Read the model definition and answer for the solid it produces. Units are mm, in the model's axes. Coordinates: 2 decimals unless noted, no trailing zeros. Write each loop counter-clockwise with the first axis right and the second up, starting at its lowest first coordinate (ties: lowest second). Pieces come first, ordered by that corner, then holes.
1) The part is cut by section B-B (x = 0.55). Determine the outline of the cut face in (y, z), then the cut area to 3 significant figures.
2) Each of these flat-tipped pins is pushed along its axis until it touches: pin 1 Ø6.5 at (y, z) = (-17, -13) entering from +X; pin 2 Ø2.5 at (y, z) = (-8, -10) entering from -X. Where does it stop, or does it pass through?
3) Find the intervals of material crossed by line 1 (Y direction, x = 0.6, z = -13); line 2 (Y direction, x = 0.2, z = 10); line 3 (Z direction, x = 0.2, y = -5), in increasing order.
4) The part is cut by section A-A (y = -17). Determine the outline of the cut face in (x, z).
from build123d import *

# Parameters (mm, degrees)
SKETCH1_W                = 36
SKETCH1_H                = 120
BOSS_EXTRUDE1_DEPTH      = 1
F_4_0_4_DIAMETER_HOLE2_D = 4
F_4_0_4_DIAMETER_HOLE3_D = 4
BOSS_EXTRUDE2_DEPTH      = 1
FILLET1_R                = 4


with BuildPart() as part:
    # Sketch1 → Boss-Extrude1 (new body)
    with BuildSketch(Plane(origin=(0, 0, 0), x_dir=(0, 0, -1), z_dir=(1, 0, 0))):
        with Locations((0, -60)):
            Rectangle(SKETCH1_W, SKETCH1_H)
    extrude(amount=BOSS_EXTRUDE1_DEPTH)

    # Ø4.0 (4) Diameter Hole2 (through all)
    with Locations(Plane.ZY):
        with Locations((-10, -8), (10, -8)):
            Hole(F_4_0_4_DIAMETER_HOLE2_D / 2)

    # Ø4.0 (4) Diameter Hole3 (through all)
    with Locations(Plane.ZY):
        with Locations((-13, -17), (13, -17)):
            Hole(F_4_0_4_DIAMETER_HOLE3_D / 2)

    # Sketch9 → Boss-Extrude2 (add)
    with BuildSketch(Plane.ZY):
        with BuildLine():
            Line((18, -23.35), (23.178427125, -28.528427125))
            ThreePointArc((23.178427125, -28.528427125), (24.04551813, -29.82612052), (24.35, -31.356854249))
            Line((24.35, -31.356854249), (24.35, -116))
            ThreePointArc((24.35, -116), (23.178427125, -118.828427125), (20.35, -120))
            Line((20.35, -120), (18, -120))
            Line((18, -120), (18, -23.35))
        make_face()
        with BuildLine():
            Line((-18, -23.35), (-23.178427125, -28.528427125))
            ThreePointArc((-23.178427125, -28.528427125), (-24.04551813, -29.82612052), (-24.35, -31.356854249))
            Line((-24.35, -31.356854249), (-24.35, -116))
            ThreePointArc((-24.35, -116), (-23.178427125, -118.828427125), (-20.35, -120))
            Line((-20.35, -120), (-18, -120))
            Line((-18, -120), (-18, -23.35))
        make_face()
    extrude(amount=-BOSS_EXTRUDE2_DEPTH)

    # Fillet1
    fillet1_edges = [part.edges().sort_by_distance(p)[0] for p in [
        (0.5, 0, 18),
        (0.5, 0, -18),
    ]]
    fillet(fillet1_edges, radius=FILLET1_R)


solid = part.part
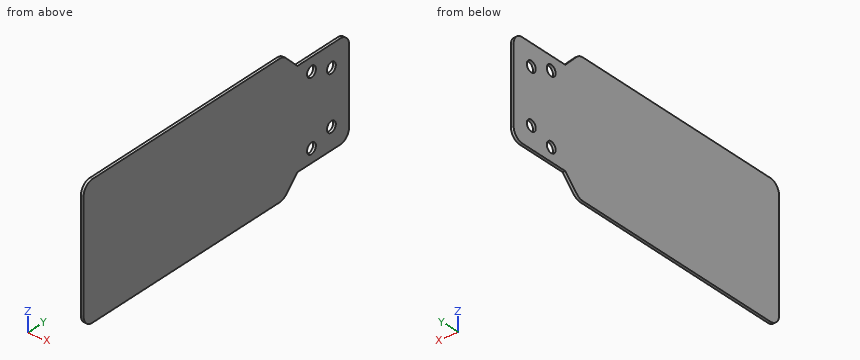
Reported:
1. outline: (-120, -20.35) arc R4 ccw to (-116, -24.35) - (-31.36, -24.35) arc R4 ccw to (-28.53, -23.18) - (-23.35, -18) - (-4, -18) arc R4 ccw to (0, -14) - (0, 14) arc R4 ccw to (-4, 18) - (-23.35, 18) - (-28.53, 23.18) arc R4 ccw to (-31.36, 24.35) - (-116, 24.35) arc R4 ccw to (-120, 20.35) - close; hole circle Ø4 at (-17, -13); hole circle Ø4 at (-17, 13); hole circle Ø4 at (-8, -10); hole circle Ø4 at (-8, 10)
1. area: 5,440 mm2
2. pin 1: stops at x = 1
2. pin 2: passes through
3. line 1: y = -120 to -19, -15 to 0
3. line 2: y = -120 to -10, -6 to 0
3. line 3: z = -18 to 18
4. outline: (0, -18) - (1, -18) - (1, -15) - (0, -15) - close; (0, -11) - (1, -11) - (1, 11) - (0, 11) - close; (0, 15) - (1, 15) - (1, 18) - (0, 18) - close
